Read the model definition and answer for the solid it produces. Units are mm, in the model's axes. Face numbers are marked on the shaded views. A direction names the side the tool comes from. Round coordinates to 2 decimals unless told otherwise and drop trailing zeros. Write each loop counter-clockwise with the first axis right and the second up, starting at its lowest first coordinate (ties: lowest second). Pieces come first, ordered by that corner, then holes. Notation, with made-up numbers: M 79.25,-33 L 93.25,-33 A8 cw 93.25,-25 Z; hole C -26.75,-8.75 d8. An arc over 180 degrees is marked long. Use one line per item in the form item = value. Start each with the question number.
```python
from build123d import *

# Parameters (mm, degrees)
SKETCH1_W           = 26.3
SKETCH1_H           = 60
SKETCH1_W_2         = 20.3
SKETCH1_H_2         = 40.3
BOSS_EXTRUDE1_DEPTH = 30
BOSS_EXTRUDE2_START = -30
SKETCH1_2_W         = 26.3
SKETCH1_2_H         = 60
BOSS_EXTRUDE2_DEPTH = 3
SKETCH2_W           = 26.3
SKETCH2_H           = 18
SKETCH2_R           = 6.575
BOSS_EXTRUDE3_DEPTH = 33
SKETCH3_W           = 10
SKETCH3_H           = 15
CUT_EXTRUDE1_DEPTH  = 20
CUT_EXTRUDE2_DEPTH  = 64.911579545
FILLET1_R           = 3
SKETCH5_R           = 2.7
CUT_EXTRUDE4_DEPTH  = 4.2
CHAMFER1_SIZE       = 0.3


with BuildPart() as part:
    # Sketch1 → Boss-Extrude1 (new body)
    with BuildSketch(Plane.XY):
        Rectangle(SKETCH1_W, SKETCH1_H)
        Rectangle(SKETCH1_W_2, SKETCH1_H_2, mode=Mode.SUBTRACT)
    extrude(amount=-BOSS_EXTRUDE1_DEPTH)

    # Sketch1<2> → Boss-Extrude2 (add)
    with BuildSketch(Plane.XY.offset(BOSS_EXTRUDE2_START)):
        Rectangle(SKETCH1_2_W, SKETCH1_2_H)
    extrude(amount=-BOSS_EXTRUDE2_DEPTH)

    # Sketch2 → Boss-Extrude3 (add)
    with BuildSketch(Plane.XY):
        with Locations((0, 39)):
            Rectangle(SKETCH2_W, SKETCH2_H)
        with Locations((0, 39)):
            Circle(SKETCH2_R, mode=Mode.SUBTRACT)
    extrude(amount=-BOSS_EXTRUDE3_DEPTH)

    # Sketch3 → Cut-Extrude1 (cut)
    with BuildSketch(Plane.XZ.offset(30)):
        with Locations((0, -25.5)):
            Rectangle(SKETCH3_W, SKETCH3_H)
    extrude(amount=-CUT_EXTRUDE1_DEPTH, mode=Mode.SUBTRACT)

    # Sketch4 → Cut-Extrude2 (cut, through all)
    with BuildSketch(Plane(origin=(13.15, 0, 0), x_dir=(0, 0, -1), z_dir=(1, 0, 0))):
        with BuildLine():
            ThreePointArc((7.4, 39), (9, 37.4), (10.6, 39))
            Line((10.6, 39), (7.4, 39))
        make_face()
        with BuildLine():
            Line((7.4, 39), (10.6, 39))
            ThreePointArc((10.6, 39), (9, 40.6), (7.4, 39))
        make_face()
        with BuildLine():
            ThreePointArc((22.4, 39), (24, 37.4), (25.6, 39))
            Line((25.6, 39), (22.4, 39))
        make_face()
        with BuildLine():
            Line((22.4, 39), (25.6, 39))
            ThreePointArc((25.6, 39), (24, 40.6), (22.4, 39))
        make_face()
    extrude(amount=-CUT_EXTRUDE2_DEPTH, mode=Mode.SUBTRACT)

    # Fillet1
    fillet1_edges = [part.edges().sort_by_distance(p)[0] for p in [
        (-13.15, 48, -16.5),
        (13.15, 48, -16.5),
        (13.15, -30, -16.5),
        (-13.15, -30, -16.5),
    ]]
    fillet(fillet1_edges, radius=FILLET1_R)

    # SurfaceCut2
    split(bisect_by=Plane.ZY, keep=Keep.TOP)

    # Sketch5 → Cut-Extrude4 (cut)
    with BuildSketch(Plane.XY):
        with Locations((-5, -25.2)):
            Circle(SKETCH5_R)
        with Locations((-5, 25.2)):
            Circle(SKETCH5_R)
    extrude(amount=-CUT_EXTRUDE4_DEPTH, mode=Mode.SUBTRACT)

    # Chamfer1
    chamfer1_edges = [part.edges().sort_by_distance(p)[0] for p in [
        (-7.7, -25.2, 0),
        (-7.7, 25.2, 0),
    ]]
    chamfer(chamfer1_edges, length=CHAMFER1_SIZE)


solid = part.part
```
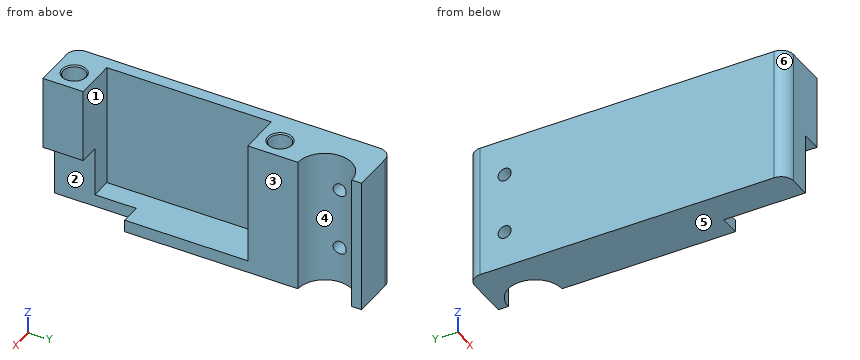
Q1. Find section B-B on x = -8.75. Write down the section's boundary in (y, z), and give its area (3 significant figures).
Q2. Each of these flat-tipped pins is pushed along its axis until it touches: pin 1 Ø4 at (y, z) = (39, -9) entering from +X; pin 2 Ø9 at (y, z) = (3.5, -17.5) entering from +X; pin 3 Ø3 at (x, y) = (-5, -25.2) entering from +Z; pin 4 Ø3 at (y, z) = (39, -24) entering from -X. Where does it stop, or does it pass through?
Q3. Find section A-A on z = -24. Write down the section's boundary in (x, y) (3 decimals).
Q4. A tool of negligible diameter and unlimited length cuts with its end or side. For the marked faces 1, 2 and 3, from which of +Z, -Z, +X, -X, +Y, -Y can it reach the whole face along a straight path? Write none if from no direction.
Q5. Straight lines are drawn through the part: line 1 (Z direction, x = -9.5, y = 39); line 2 (Y direction, x = -9.25, z = -9); line 3 (Y direction, x = -7, z = -12). For each, find the intervals that lie inside material, in ascending order. Write a range as [from, to].
Q6. Find section D-D on y = -25.2. Write down the section's boundary in (x, z).
Q7. For a pull along Y with two mould halves and no side action, classify the marked faces 4, 5 and 6 as +Y half, -Y half, draft (parallel to the pull), parting line (faces both ways), or undercut.
Q8. Find section C-C on y = 39. Write down the section's boundary in (x, z) (3 decimals).
Response:
q1.outline = M -30,-33 L 48,-33 L 48,0 L 20.15,0 L 20.15,-30 L -20.15,-30 L -20.15,0 L -30,0 Z; hole C 39,-24 d3.2; hole C 39,-9 d3.2
q1.area = 1,350 mm²
q2.pin_1 = -6.26
q2.pin_2 = -10.15
q2.pin_3 = -4.2
q2.pin_4 = through
q3.outline = M -13.15,-27 A3 ccw -10.15,-30 L -5,-30 L -5,-20.15 L -10.15,-20.15 L -10.15,20.15 L 0,20.15 L 0,32.425 A6.575 cw -6.377,37.4 L -13.15,37.4 Z; M -13.15,40.6 L -6.377,40.6 A6.575 cw 0,45.575 L 0,48 L -10.15,48 A3 ccw -13.15,45 Z
q4.face_1 = +Z, +X
q4.face_2 = -Z, +X, -Y
q4.face_3 = +Z, -Z, +X, +Y, -Y
q5.line_1 = [-33, -25.6], [-22.4, -10.6], [-7.4, 0]
q5.line_2 = [-30, -20.15], [20.15, 37.4], [40.6, 48]
q5.line_3 = [-30, -20.15], [20.15, 48]
q6.outline = M -13.15,-33 L -5,-33 L -5,-18 L 0,-18 L 0,0 L -2,0 L -2.3,-0.3 L -2.3,-4.2 L -7.7,-4.2 L -7.7,-0.3 L -8,0 L -13.15,0 Z
q7.face_4 = undercut
q7.face_5 = draft
q7.face_6 = -Y half
q8.outline = M -13.15,-33 L -6.575,-33 L -6.575,-25.6 L -13.15,-25.6 Z; M -13.15,-22.4 L -6.575,-22.4 L -6.575,-10.6 L -13.15,-10.6 Z; M -13.15,-7.4 L -6.575,-7.4 L -6.575,0 L -13.15,0 Z
